Autodesk Fusion 360 part; units mm, degrees
sketch "Sketch1" plane through (0, 0, 0) normal (0, 0, 1) x (1, 0, 0)
  line L0 (35.5, 35.5) -> (-35.5, 35.5) construction
  line L1 (-35.5, 35.5) -> (-35.5, -35.5) construction
  line L2 (-35.5, -35.5) -> (35.5, -35.5) construction
  line L3 (35.5, -35.5) -> (35.5, 35.5) construction
  line L4 (35.5, 35.5) -> (-35.5, -35.5) construction
  line L5 (-35.5, 35.5) -> (35.5, -35.5) construction
  circle A0 centre (-35.5, 35.5) radius 2.5
  circle A1 centre (35.5, 35.5) radius 2.5
  circle A2 centre (-35.5, -35.5) radius 2.5
  circle A3 centre (35.5, -35.5) radius 2.5
  line L6 (63, 50) -> (-63, 50) construction
  line L7 (-63, 50) -> (-63, -50) construction
  line L8 (-63, -50) -> (63, -50) construction
  line L9 (63, -50) -> (63, 50) construction
  line L10 (63, 50) -> (-63, -50) construction
  line L11 (-63, 50) -> (63, -50) construction
  line L12 (40, 40) -> (-40, 40) construction
  line L13 (-40, 40) -> (-40, -40) construction
  line L14 (-40, -40) -> (40, -40) construction
  line L15 (40, -40) -> (40, 40) construction
  line L16 (40, 40) -> (-40, -40) construction
  line L17 (-40, 40) -> (40, -40) construction
  line L18 (-22.5, 40) -> (-40, 22.5)
  line L19 (0, 0) -> (0, 35.5) construction
  line L20 (0, 0) -> (35.5, 0) construction
  line L21 (22.5, 40) -> (40, 22.5)
  line L22 (-22.5, -40) -> (-40, -22.5)
  line L23 (22.5, -40) -> (40, -22.5)
  line L24 (-40, -22.5) -> (-40, 22.5)
  line L25 (-22.5, 40) -> (22.5, 40)
  line L26 (40, 22.5) -> (40, -22.5)
  line L27 (-22.5, -40) -> (22.5, -40)
  circle A4 centre (-70, 3) radius 3
  circle A5 centre (-70, 38) radius 3
  circle A6 centre (70, 38) radius 3
  circle A7 centre (70, 3) radius 3
  line L28 (-70, 38) -> (-70, 3) construction
  circle A8 centre (-70, 20.5) radius 2.5
  circle A9 centre (70, 20.5) radius 2.5
  line L29 (-72, -50) -> (72, -50)
  line L30 (82, -40) -> (82, 40)
  line L31 (72, 50) -> (-72, 50)
  line L32 (-82, 40) -> (-82, -40)
  arc A10 (-72, 50) -> (-82, 40) centre (-72, 40) ccw
  arc A11 (82, 40) -> (72, 50) centre (72, 40) ccw
  arc A12 (72, -50) -> (82, -40) centre (72, -40) ccw
  arc A13 (-82, -40) -> (-72, -50) centre (-72, -40) ccw
  point P0 (-70, 38)
  point P1 (-82, -50)
  point P2 (82, -50)
  point P3 (82, 50)
  dimension "d1" = 71
  dimension "d2" = 71
  dimension "d3" = 5
  dimension "d4" = 5
  dimension "d5" = 5
  dimension "d6" = 5
  dimension "d7" = 126
  dimension "d8" = 100
  dimension "d9" = 80
  dimension "d10" = 80
  dimension "d11" = 13
  dimension "d12" = 45
  dimension "d13" = 12
  dimension "d14" = 70
  dimension "d15" = 5
  dimension "d16" = 12
  dimension "d17" = 10
extrude "Extrude1" add sketch "Sketch1" along normal blind 3
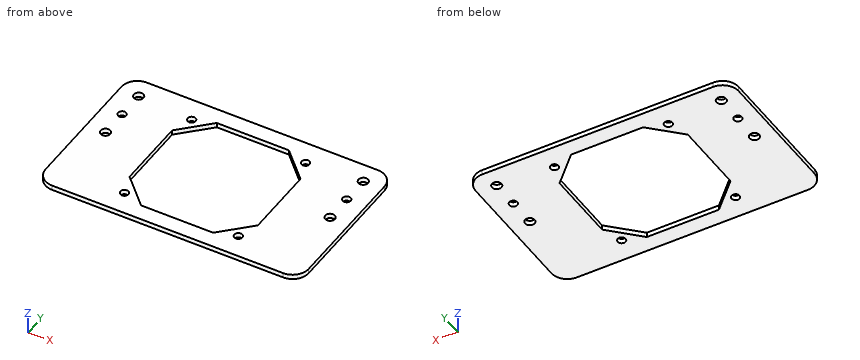
CAD build for the part. Positions are in the model's coordinates, mm. Round coordinates to 2 decimals unless told otherwise and drop trailing zeros. Loops run counter-clockwise (first coordinate to the right, second up) from the corner with the lowest first, then second, coordinate; pieces in that order, holes last. Notation, with made-up numbers: (70.25, 5) - (115.25, 5) arc R30 ccw to (115.25, 38) - close; hole circle Ø5 at (74.25, 77). An arc over 180 degrees is marked (long way). Return JSON: item names as keys, results as strings. Group by question number.
Q1. Band-saw the part on A-A on x = 35.5. Give the cut face in (y, z), plus the area to 3 significant figures.
Q2. Drill centre lines: line 1 along Y through (x, z) = (-70, 1.55); line 2 along Y through (x, z) = (37, 2.75); line 3 along Y through (x, z) = (10.5, 1.9). Where is each one in solid material? Low to high. Write a range as [from, to].
Q3. Band-saw the part on B-B on y = 3. Give the cut face in (x, z), plus the area to 3 significant figures.
Q4. Band-saw the part on D-D on y = -12.5. Give the cut face in (x, z).
Q5. Flat gauge pin, fed straight in: pin 1 Ø3 at (x, y) = (-35.5, -35.5) entering from -Z. Where does the tip first touch, or does it go through?
Q6. Band-saw the part on C-C on x = -3. Give the cut face in (y, z).
Solutions:
{
 "1": {"outline": "(-50, 0) - (-38, 0) - (-38, 3) - (-50, 3) - close; (-33, 0) - (-27, 0) - (-27, 3) - (-33, 3) - close; (27, 0) - (33, 0) - (33, 3) - (27, 3) - close; (38, 0) - (50, 0) - (50, 3) - (38, 3) - close", "area": "108 mm^2"},
 "2": {"line 1": "y = [-50, 0], [6, 18], [23, 35], [41, 50]", "line 2": "y = [-50, -37.5], [-33.5, -25.5], [25.5, 33.5], [37.5, 50]", "line 3": "y = [-50, -40], [40, 50]"},
 "3": {"outline": "(-82, 0) - (-73, 0) - (-73, 3) - (-82, 3) - close; (-67, 0) - (-40, 0) - (-40, 3) - (-67, 3) - close; (40, 0) - (67, 0) - (67, 3) - (40, 3) - close; (73, 0) - (82, 0) - (82, 3) - (73, 3) - close", "area": "216 mm^2"},
 "4": {"outline": "(-82, 0) - (-40, 0) - (-40, 3) - (-82, 3) - close; (40, 0) - (82, 0) - (82, 3) - (40, 3) - close"},
 "5": {"pin 1": "passes through"},
 "6": {"outline": "(-50, 0) - (-40, 0) - (-40, 3) - (-50, 3) - close; (40, 0) - (50, 0) - (50, 3) - (40, 3) - close"}
}
